Check sheet for the modelled part. Datum: model origin and axes. Units: mm. Face numbers are marked on the shaded views. A direction names the side the tool comes from. Coordinates: 2 decimals unless noted, no trailing zeros. Write each loop counter-clockwise with the first axis right and the second up, starting at its lowest first coordinate (ties: lowest second). Pieces come first, ordered by that corner, then holes. Notation, with made-up numbers: (31, -23) -> (79, -23) arc R28 ccw to (79, -2) -> close; hole circle Ø10 at (-11, -17). An arc over 180 degrees is marked (long way). One line per item, written item: value. Start each with the question number.
1) Draft check along Z on the marked faces 1, 2 and 3. Enter one of: +Z half, -Z half, draft (parallel to the pull), parting line (faces both ways), or undercut.
2) Sectioned sample at A-A on y = 187. Enter the section's corners in (x, z), plus the area to 3 significant figures.
3) Sectioned sample at D-D on x = -165. Enter the section's corners in (y, z).
4) Sectioned sample at C-C on x = -83. Enter the section's corners in (y, z), plus the area to 3 significant figures.
5) Set-up check for the marked faces 4, 5 and 6: record each of +Z, -Z, +X, -X, +Y, -Y from which the full face is reachable in a straight line by a thin tool's end or side.
6) Scan lines: line 1 along Z through (x, y) = (-138.5, 420); line 2 along X through (y, z) = (139, 489); line 3 along X through (y, z) = (407, 422). Record each from-to range of solid material in increasing order. Write a range as [from, to].
7) Gauge pin test, flat ends, axial feed: P1, Ø1.5, axis at y = 263.5, z = -82.5, coming from the +X side; P2, Ø1.5, axis at x = -160, z = -292, coming from the +Y side; P3, Ø4, axis at x = -186, z = 63.5, coming from the -Y side. Record the tip position at first contact, or that the pin passes through.
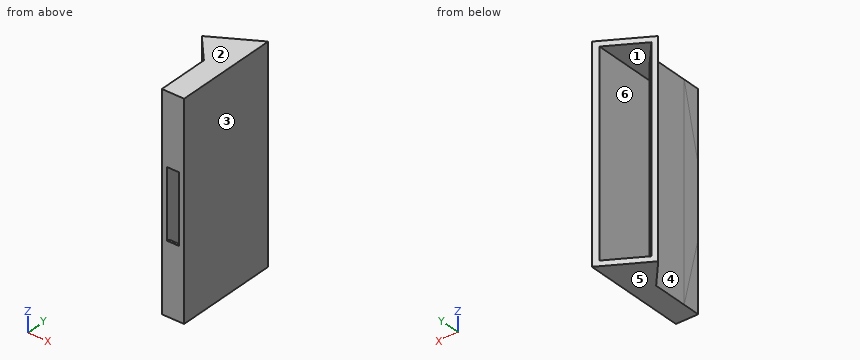
```python
from build123d import *

# Parameters (mm, degrees)
BOSS_EXTRUDE1_DEPTH = 600
SHELL1_T            = -30
SKETCH3_W           = 67.520055582
SKETCH3_H           = 1140
CUT_EXTRUDE1_DEPTH  = 806.232885568
BOSS_EXTRUDE2_DEPTH = 127.52006
SHELL2_START        = -97.520055582
SHELL2_DEPTH        = 67.520055582
SKETCH5_W           = 67.520055582
SKETCH5_H           = 392.613662462
CUT_EXTRUDE2_DEPTH  = 868.409937688
BOSS_EXTRUDE3_DEPTH = 127.520055582
FILLET1_R           = 40


# Read off the part's stored shape, not the designer's step: Shell2
with BuildPart() as part:
    # Sketch2 → Boss-Extrude1 (new, symmetric)
    with BuildSketch(Plane.XY):
        Polygon((0, 0), (0, 500), (-259.807621135, 350), (-127.520055582, 200), (-127.520055582, 0), align=None)
    extrude(amount=BOSS_EXTRUDE1_DEPTH, both=True)

    # Shell1
    shell1_openings = [part.faces().sort_by_distance(p)[0] for p in [
        (-129.903810568, 425, 0),
    ]]
    offset(amount=SHELL1_T, openings=shell1_openings, kind=Kind.INTERSECTION)

    # Sketch3 → Cut-Extrude1 (cut, through all)
    with BuildSketch(Plane(origin=(0, 30, 0), x_dir=(1, 0, 0), z_dir=(0, 1, 0))):
        with Locations((-63.760027791, 0)):
            Rectangle(SKETCH3_W, SKETCH3_H)
    extrude(amount=-CUT_EXTRUDE1_DEPTH, mode=Mode.SUBTRACT)

    # Sketch4 → Boss-Extrude2 (add)
    with BuildSketch(Plane(origin=(0, 0, 0), x_dir=(0, 0, -1), z_dir=(1, 0, 0))):
        Polygon((-600, 0), (600, 0), (200, -100), (-200, -100), align=None)
    extrude(amount=-BOSS_EXTRUDE2_DEPTH)

    # Shell2 outline → Shell2 (cut)
    with BuildSketch(Plane.YZ.offset(SHELL2_START)):
        Polygon((0, -476.306831231), (0, 476.306831231), (-70, 196.306831231), (-70, -196.306831231), align=None)
    extrude(amount=SHELL2_DEPTH, mode=Mode.SUBTRACT)

    # Sketch5 → Cut-Extrude2 (cut, through all)
    with BuildSketch(Plane(origin=(0, -70, 0), x_dir=(1, 0, 0), z_dir=(0, 1, 0))):
        with Locations((-63.760027791, 0)):
            Rectangle(SKETCH5_W, SKETCH5_H)
    extrude(amount=-CUT_EXTRUDE2_DEPTH, mode=Mode.SUBTRACT)

    # Sketch6 → Boss-Extrude3 (add)
    with BuildSketch(Plane(origin=(0, 0, -600), x_dir=(0, 0, -1), z_dir=(1, 0, 0))):
        Polygon((-1200, 0), (-800, -100), (-1200, -100), align=None)
        Polygon((-400, -100), (0, 0), (0, -100), align=None)
    extrude(amount=-BOSS_EXTRUDE3_DEPTH)

    # Fillet1
    # the kernel refuses this fillet: 40 mm, written as the material it takes off along each edge
    with BuildSketch(Plane(origin=(-97.520055582, -70, 196.306831231), x_dir=(0, 0.24253562503633297, 0.9701425001453319), z_dir=(1, 0, 0))) as fillet1_piece_1:
        with BuildLine():
            CenterArc((31.211373056, 40), FILLET1_R, 195.806721483, 74.193278517)
            Line((-7.276068751, 29.104275004), (0, 0))
            Line((0, 0), (31.211373056, 0))
        make_face()
    extrude(amount=67.520055582, mode=Mode.SUBTRACT)
    with BuildSketch(Plane(origin=(-97.520055582, -70, -196.306831231), x_dir=(0, 0.24253562503633297, -0.9701425001453319), z_dir=(1, 0, 0))) as fillet1_piece_2:
        with BuildLine():
            CenterArc((31.211373056, -40), FILLET1_R, 90, 74.193278517)
            Line((-7.276068751, -29.104275004), (0, 0))
            Line((0, 0), (31.211373056, 0))
        make_face()
    extrude(amount=67.520055582, mode=Mode.SUBTRACT)


solid = part.part
```
Answers:
1. face 1: undercut
1. face 2: +Z half
1. face 3: draft
2. outline: (-127.52, -600) -> (0, -600) -> (0, 600) -> (-127.52, 600) -> close; hole (-97.52, -570) -> (-30, -570) -> (-30, 570) -> (-97.52, 570) -> close
2. area: 76,100 mm2
3. outline: (242.5, -600) -> (404.74, -600) -> (404.74, -570) -> (287.85, -570) -> (287.85, 570) -> (404.74, 570) -> (404.74, 600) -> (242.5, 600) -> close
4. outline: (-100, -600) -> (452.08, -600) -> (452.08, -570) -> (0, -570) -> (0, -476.31) -> (-62.43, -226.59) arc R40 ccw to (-100, -196.31) -> close; (-100, 196.31) arc R40 ccw to (-62.43, 226.59) -> (0, 476.31) -> (0, 570) -> (452.08, 570) -> (452.08, 600) -> (-100, 600) -> close
4. area: 87,900 mm2
5. face 4: +Z, -Z, -X, -Y
5. face 5: -Z, +X, -X, +Y, -Y
5. face 6: +Y
6. line 1: z = [-600, -570], [570, 600]
6. line 2: x = [-127.52, -97.52], [-30, 0]
6. line 3: x = [-30, 0]
7. P1: stops at x = 0
7. P2: stops at y = 283.03
7. P3: stops at y = 264.04
